Drawing for the job (mm, zero at the part's lowest x, y, z). A direction names the side the tool comes from. Give positions to 0.01 mm unless a question says otherwise; leave off trailing zeros. Write each loop counter-clockwise with the first axis right and the second up, starting at its lowest first coordinate (ties: lowest second). Pieces come first, ordered by that corner, then holes. Notation, with made-up numbers: (2, 21) - (6, 21) arc R16 ccw to (6, 42) - close; hole circle Ø3 at (65.5, -27). An arc over 180 degrees is marked (long way). Use CSV: the item, a comma, the result in double quotes.
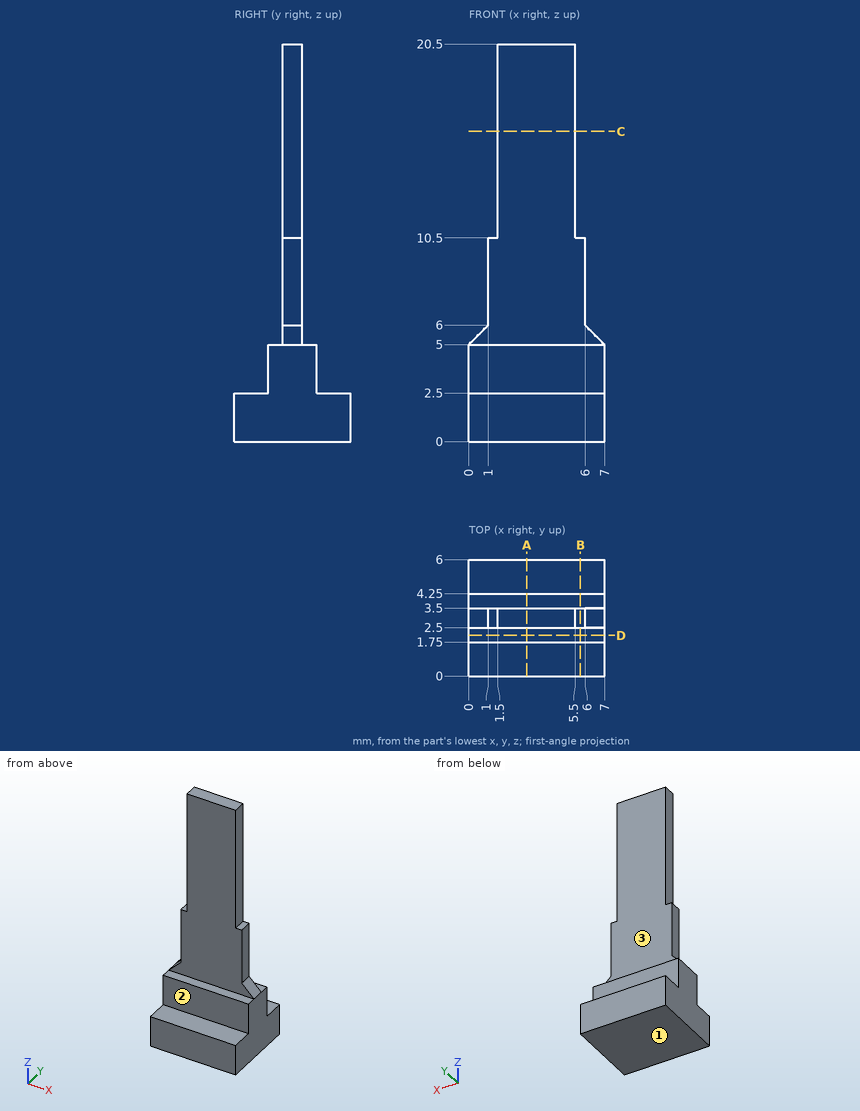
(1) 3-axis set-ups, long thin cutter, end or side, ignore diameter. For the marked faces 1, 2 and 3: which of +Z, -Z, +X, -X, +Y, -Y reach the whole face in a straight line?
Checked values:
face 1,"-Z, +X, -X, +Y, -Y"
face 2,"+Z, +X, -X, -Y"
face 3,"+Z, +X, -X, +Y"
(2) Saw through at C-C, the plane z = 16. List the corners of the cut face in (x, y), then the cut area to 3 significant figures.
Checked values:
outline,"(1.5, 2.5) - (5.5, 2.5) - (5.5, 3.5) - (1.5, 3.5) - close"
area,"4.00 mm^2"
(3) Saw through at B-B, the plane x = 5.75. List the corners of the cut face in (y, z).
Checked values:
outline,"(0, 0) - (6, 0) - (6, 2.5) - (4.25, 2.5) - (4.25, 5) - (3.5, 5) - (3.5, 10.5) - (2.5, 10.5) - (2.5, 5) - (1.75, 5) - (1.75, 2.5) - (0, 2.5) - close"
(4) Flat gauge pins, fed straight in: P1, Ø2, axis at x = 1.5, z = 11.5, coming from the -Y side; P2, Ø1.4, axis at x = 3, y = 5.5, coming from the +Z side; P3, Ø2, axis at x = 3, z = 13.5, coming from the +Y side. Where does each tip first touch, or does it go through?
Checked values:
P1,"stops at y = 2.5"
P2,"stops at z = 2.5"
P3,"stops at y = 3.5"
(5) Saw through at A-A, the plane x = 3. List the corners of the cut face in (y, z).
Checked values:
outline,"(0, 0) - (6, 0) - (6, 2.5) - (4.25, 2.5) - (4.25, 5) - (3.5, 5) - (3.5, 20.5) - (2.5, 20.5) - (2.5, 5) - (1.75, 5) - (1.75, 2.5) - (0, 2.5) - close"
(6) Saw through at D-D, the plane y = 2.1. List the corners of the cut face in (x, z).
Checked values:
outline,"(0, 0) - (7, 0) - (7, 5) - (0, 5) - close"
(7) Wall check: probe 1 along Y at (x, z) = (4.75, 11.75); probe 2 along Z at (x, y) = (2.75, 4); probe 3 along Z at (x, y) = (3.25, 5.25). Give the ranges that are in metal, low to high. Write a range as [from, to].
Checked values:
probe 1,"y = [2.5, 3.5]"
probe 2,"z = [0, 5]"
probe 3,"z = [0, 2.5]"
